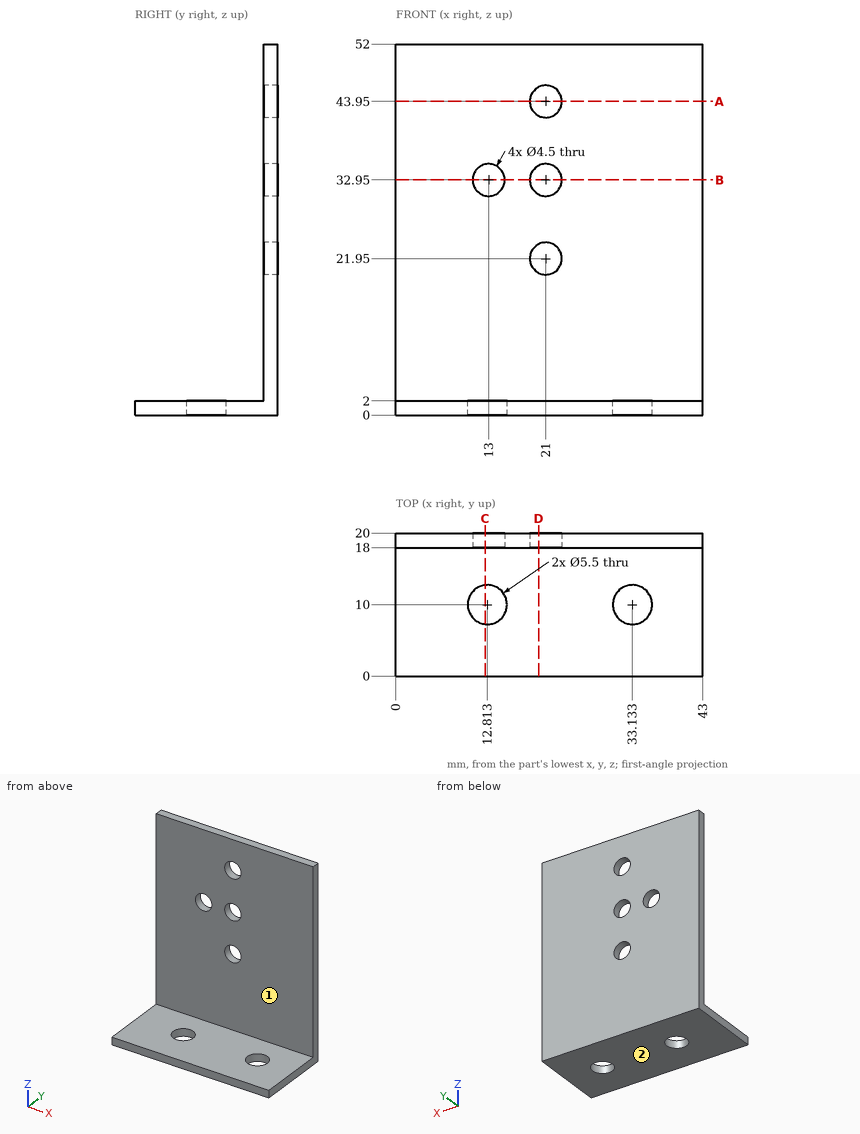
Could you check a few things on this drawing? It's one solid part, dimensions in mm from its lowest x, y, z. A direction names the side the tool comes from. Give positions to 0.01 mm unless a question says otherwise; leave off trailing zeros. Write each loop counter-clockwise with the first axis right and the second up, starting at its lowest first coordinate (ties: lowest second). Pieces come first, ordered by that corner, then holes. Notation, with made-up numbers: (81, 34) -> (114, 34) arc R18 cw to (114, 44) -> close; hole circle Ø6 at (26.25, -1). An arc over 180 degrees is marked (long way). Answer as a JSON object with one key per item and string values.
Q1. Suppose I cut it at B-B on z = 32.95. Write out the boundary of the cut face in (x, y).
Taken from the geometry:
{"outline": "(0, 18) -> (10.75, 18) -> (10.75, 20) -> (0, 20) -> close; (15.25, 18) -> (18.75, 18) -> (18.75, 20) -> (15.25, 20) -> close; (23.25, 18) -> (43, 18) -> (43, 20) -> (23.25, 20) -> close"}
Q2. Which directions (+Z, -Z, +X, -X, +Y, -Y) give clear straight access to the entire face, cutting with the end or side of a thin tool? Please do the marked faces 1 and 2.
Taken from the geometry:
{"face 1": "+Z, +X, -X, -Y", "face 2": "-Z, +X, -X, +Y, -Y"}
Q3. Will these pins go through, and if not, where does the flat tip stop? pin 1 Ø5 at (x, z) = (21, 32.95) entering from -Y; pin 2 Ø3.5 at (x, z) = (21, 21.95) entering from -Y; pin 3 Ø4 at (x, y) = (37.5, 5) entering from +Z.
Taken from the geometry:
{"pin 1": "stops at y = 18", "pin 2": "passes through", "pin 3": "stops at z = 2"}
Q4. Please list where these lines run through material, in increasing order: L1, parallel to X at y = 19.1, z = 32.95; L2, parallel to Z at x = 21, y = 18.95; L3, parallel to Z at x = 13, y = 19.2.
Taken from the geometry:
{"L1": "x = 0 to 10.75, 15.25 to 18.75, 23.25 to 43", "L2": "z = 0 to 19.7, 24.2 to 30.7, 35.2 to 41.7, 46.2 to 52", "L3": "z = 0 to 30.7, 35.2 to 52"}
Q5. Suppose I cut it at C-C on x = 12.5. Write out the boundary of the cut face in (y, z), then the cut area to 3 significant figures.
Taken from the geometry:
{"outline": "(0, 0) -> (7.27, 0) -> (7.27, 2) -> (0, 2) -> close; (12.73, 0) -> (20, 0) -> (20, 30.76) -> (18, 30.76) -> (18, 2) -> (12.73, 2) -> close; (18, 35.14) -> (20, 35.14) -> (20, 52) -> (18, 52) -> close", "area": "120 mm²"}
Q6. Suppose I cut it at D-D on x = 20. Write out the boundary of the cut face in (y, z) (1 decimal).
Taken from the geometry:
{"outline": "(0, 0) -> (20, 0) -> (20, 19.9) -> (18, 19.9) -> (18, 2) -> (0, 2) -> close; (18, 24) -> (20, 24) -> (20, 30.9) -> (18, 30.9) -> close; (18, 35) -> (20, 35) -> (20, 41.9) -> (18, 41.9) -> close; (18, 46) -> (20, 46) -> (20, 52) -> (18, 52) -> close"}
Q7. Suppose I cut it at A-A on z = 43.95. Write out the boundary of the cut face in (x, y).
Taken from the geometry:
{"outline": "(0, 18) -> (18.75, 18) -> (18.75, 20) -> (0, 20) -> close; (23.25, 18) -> (43, 18) -> (43, 20) -> (23.25, 20) -> close"}
